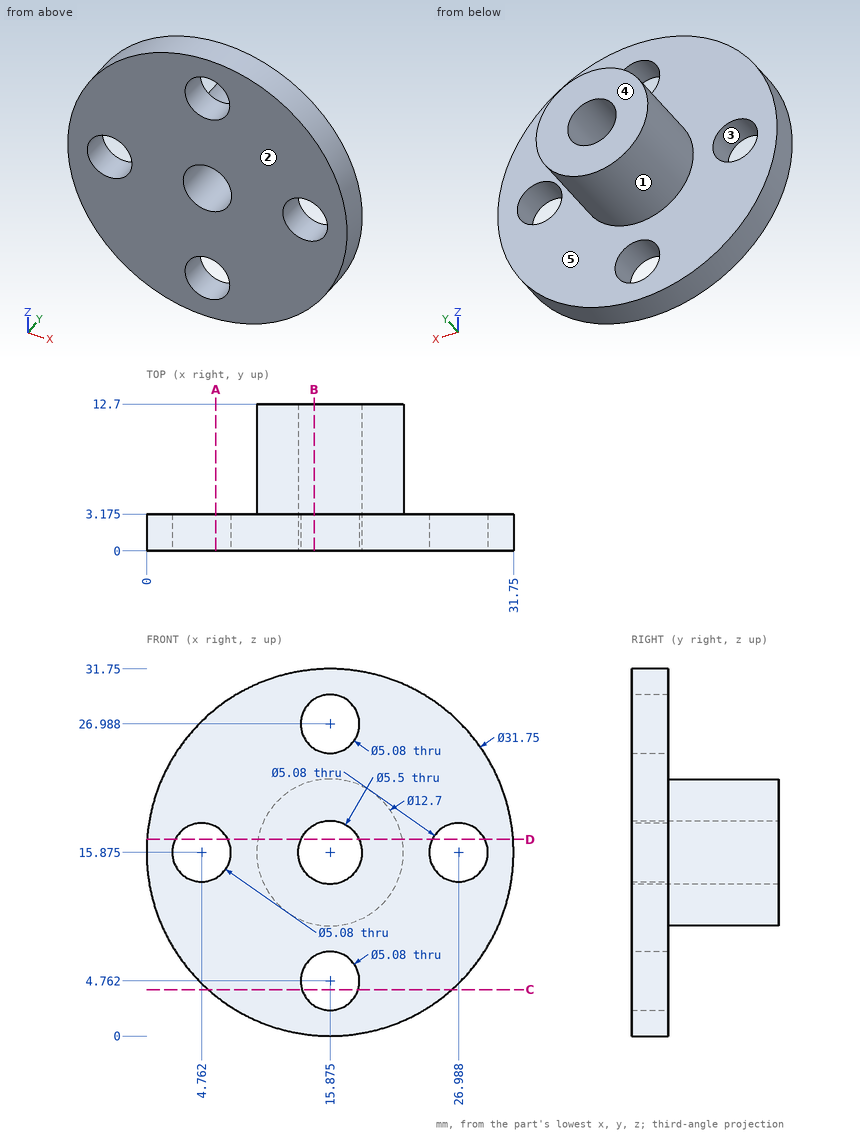
Could you check a few things on this drawing? It's one solid part, dimensions in mm from its lowest x, y, z. A direction names the side the tool comes from. Coordinates: 2 decimals unless noted, no trailing zeros. Loops run counter-clockwise (first coordinate to the right, second up) from the corner with the lowest first, then second, coordinate; pieces in that order, holes last.
1. For P1, Ø2, axis at y = 3.5, z = 18.5, coming from the -X side; P2, Ø2, axis at y = 2, z = 24.5, coming from the -X side; P3, Ø8, axis at x = 15.88, z = 26.99, coming from the +Y side (1 decimal), each with a flat end and sliding along its axis, tell me the tip position at first contact or that it passes through.
2. I need wall thicknesses on L1, parallel to Z at x = 16, y = 6.25; L2, parallel to Z at x = 17.5, y = 11 (1 decimal); L3, parallel to Y at x = 25, z = 10.5 (1 decimal). Which ranges of each line are inside material? Lowest first, please.
3. Imagine slicing it at C-C (z = 4). Please give me the cut outline in (x, y) (1 decimal).
4. Imagine slicing it at B-B (x = 14.5). Please give me the cut outline in (y, z) (1 decimal), and give its area (3 significant figures).
5. Imagine slicing it at A-A (x = 6). Please give me the cut outline in (y, z) (1 decimal).
6. Imagine slicing it at D-D (z = 17). Please give me the cut outline in (x, y) (1 decimal), and give its area (3 significant figures).
7. We'd pull the mould along Z, two halves only. Please class the marked faces 1, 2 and 3: released by +Z, released by -Z, zero draft, split by the parting line, or undercut.
8. For the marked faces 4 and 5, which set-ups out of +Z, -Z, +X, -X, +Y, -Y let a thin tool reach every point of the face, with its end or its side?
Computed values:
1. P1: stops at x = 0.09
1. P2: stops at x = 1.95
1. P3: stops at y = 3.2
2. L1: z = 9.53 to 13.13, 18.62 to 22.22
2. L2: z = 9.7 to 13.7, 18.1 to 22
2. L3: y = 0 to 3.2
3. outline: (5.3, 0) - (13.5, 0) - (13.5, 3.2) - (5.3, 3.2) - close; (18.3, 0) - (26.4, 0) - (26.4, 3.2) - (18.3, 3.2) - close
4. outline: (0, 0.1) - (3.2, 0.1) - (3.2, 2.6) - (0, 2.6) - close; (0, 6.9) - (3.2, 6.9) - (3.2, 9.7) - (12.7, 9.7) - (12.7, 13.5) - (0, 13.5) - close; (0, 18.3) - (12.7, 18.3) - (12.7, 22.1) - (3.2, 22.1) - (3.2, 24.9) - (0, 24.9) - close; (0, 29.1) - (3.2, 29.1) - (3.2, 31.7) - (0, 31.7) - close
4. area: 131 mm2
5. outline: (0, 3.4) - (3.2, 3.4) - (3.2, 13.7) - (0, 13.7) - close; (0, 18.1) - (3.2, 18.1) - (3.2, 28.3) - (0, 28.3) - close
6. outline: (0, 0) - (2.5, 0) - (2.5, 3.2) - (0, 3.2) - close; (7, 0) - (13.4, 0) - (13.4, 12.7) - (9.6, 12.7) - (9.6, 3.2) - (7, 3.2) - close; (18.4, 0) - (24.7, 0) - (24.7, 3.2) - (22.1, 3.2) - (22.1, 12.7) - (18.4, 12.7) - close; (29.3, 0) - (31.7, 0) - (31.7, 3.2) - (29.3, 3.2) - close
6. area: 127 mm2
7. face 1: split by the parting line
7. face 2: zero draft
7. face 3: undercut
8. face 4: +Z, -Z, +X, -X, +Y
8. face 5: +Y
